Could you check a few things on this model? Use its own coordinates, in mm. Face numbers are marked on the shaded views. A direction names the side the tool comes from. Round coordinates to 2 decimals unless told otherwise and drop trailing zeros. Order: outer loops, then holes, each group sorted by start corner. A loop starts at its lowest first (then second) coordinate and runs counter-clockwise, first axis right, second up. Notation, with made-up numbers: (44, -2) - (58, -2) arc R27 ccw to (58, 33) - close; hole circle Ø7 at (30, 66). An arc over 180 degrees is marked (long way). Return JSON: item names as keys, results as strings. Group by question number.
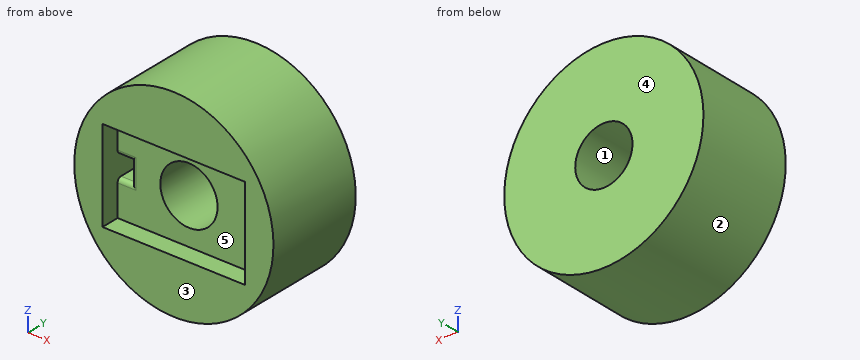
from build123d import *

# Parameters (mm, degrees)
SKETCH3_R           = 12
BOSS_EXTRUDE1_DEPTH = 12
SKETCH2_W           = 17.2
SKETCH2_H           = 11
CUT_EXTRUDE1_DEPTH  = 2.2
SKETCH4_R           = 3.45
CUT_EXTRUDE2_DEPTH  = 21.784609691
SKETCH5_W           = 1.698676218
SKETCH5_H           = 2.5
CUT_EXTRUDE3_DEPTH  = 2.5
FILLET1_R           = 0.5


with BuildPart() as part:
    # Sketch3 → Boss-Extrude1 (new body)
    with BuildSketch(Plane(origin=(0, 0, 0), x_dir=(1, 0, 0), z_dir=(0, 1, 0))):
        with Locations(Location((0, 0, 0), (0, 0, 270))):
            Circle(SKETCH3_R)
    extrude(amount=BOSS_EXTRUDE1_DEPTH)

    # Sketch2 → Cut-Extrude1 (cut)
    with BuildSketch(Plane(origin=(0, 0, 0), x_dir=(1, 0, 0), z_dir=(0, 1, 0))):
        Rectangle(SKETCH2_W, SKETCH2_H)
    extrude(amount=CUT_EXTRUDE1_DEPTH, mode=Mode.SUBTRACT)

    # Sketch4 → Cut-Extrude2 (cut, through all)
    with BuildSketch(Plane(origin=(0, 0, 0), x_dir=(1, 0, 0), z_dir=(0, 1, 0))):
        with Locations(Location((0, 0, 0), (0, 0, 90))):
            Circle(SKETCH4_R)
    extrude(amount=CUT_EXTRUDE2_DEPTH, mode=Mode.SUBTRACT)

    # Sketch5 → Cut-Extrude3 (cut)
    with BuildSketch(Plane.XZ.offset(-2.2)):
        with Locations((-7.750661891, 0)):
            Rectangle(SKETCH5_W, SKETCH5_H)
    extrude(amount=-CUT_EXTRUDE3_DEPTH, mode=Mode.SUBTRACT)

    # Fillet1
    fillet1_edges = [part.edges().sort_by_distance(p)[0] for p in [
        (-7.750661891, 2.2, -1.25),
        (-6.901323782, 2.2, 0),
        (-7.750661891, 2.2, 1.25),
    ]]
    fillet(fillet1_edges, radius=FILLET1_R)


solid = part.part
1) If I drill on line 1 along X through (y, z) = (9.75, 0); line 2 along Y through (x, z) = (8, 1.75); line 3 along X through (y, z) = (11, -1.5), over which ranges is the centre line in solid material (lowest first)? Write a range as from..to.
2) For the marked faces 4 and 5, which set-ups out of +Z, -Z, +X, -X, +Y, -Y let a thin tool reach every point of the face, with its end or its side?
3) I want a section at B-B, the plane y = 4. List the corners of the cut face in (x, z) for me.
4) We'd pull the mould along X, two halves only. Please class the marked faces 1, 2 and 3: +X half, -X half, draft (parallel to the pull), parting line (faces both ways), or undercut.
5) Will these pins go through, and if not, where does the flat tip stop? pin 1 (8 mm diameter, centred on x = 3.5, z = -3.5, fed in from -Y); pin 2 (3 mm diameter, centred on x = 3, y = 10.5, fed in from -Z); pin 3 (9 mm diameter, centred on x = -2, z = -0.5, fed in from -Y); pin 4 (0.7 mm diameter, centred on x = 1, y = 1.5, fed in from +Z).
6) I want a section at C-C, the plane x = -0.75. List the corners of the cut face in (y, z) for me, plus the area to 3 significant figures.
7) I want a section at A-A, the plane z = 0. List the corners of the cut face in (x, y) for me.
8) I want a section at D-D, the plane x = 4. List the corners of the cut face in (y, z) for me, plus the area to 3 significant figures.
Outcome:
{
 "1": {"line 1": "-12..-3.45, 3.45..12", "line 2": "2.2..12", "line 3": "-11.91..-3.11, 3.11..11.91"},
 "2": {"face 4": "+Z, -Z, +X, -X, +Y", "face 5": "-Y"},
 "3": {"outline": "circle Ø24 at (0, 0); hole (-8.6, -1.25) - (-6.9, -1.25) - (-6.9, 1.25) - (-8.6, 1.25) - close; hole circle Ø6.9 at (0, 0)"},
 "4": {"face 1": "undercut", "face 2": "parting line", "face 3": "draft"},
 "5": {"pin 1": "y = 0", "pin 2": "z = -11.91", "pin 3": "y = 2.2", "pin 4": "z = 11.98"},
 "6": {"outline": "(0, -11.98) - (12, -11.98) - (12, -3.37) - (2.2, -3.37) - (2.2, -5.5) - (0, -5.5) - close; (0, 5.5) - (2.2, 5.5) - (2.2, 3.37) - (12, 3.37) - (12, 11.98) - (0, 11.98) - close", "area": "197 mm^2"},
 "7": {"outline": "(-12, 0) - (-8.6, 0) - (-8.6, 4.7) - (-6.9, 4.7) - (-6.9, 2.7) arc R0.5 ccw to (-6.4, 2.2) - (-3.45, 2.2) - (-3.45, 12) - (-12, 12) - close; (3.45, 2.2) - (8.6, 2.2) - (8.6, 0) - (12, 0) - (12, 12) - (3.45, 12) - close"},
 "8": {"outline": "(0, -11.31) - (12, -11.31) - (12, 11.31) - (0, 11.31) - (0, 5.5) - (2.2, 5.5) - (2.2, -5.5) - (0, -5.5) - close", "area": "247 mm^2"}
}
